```python
from build123d import *

# Parameters (mm, degrees)
SKETCH1_R           = 57.5
BOSS_EXTRUDE1_DEPTH = 4.5
SKETCH2_W           = 140
SKETCH2_H           = 70
BOSS_EXTRUDE2_DEPTH = 4.5
BOSS_EXTRUDE3_DEPTH = 4.5
SKETCH4_R           = 43
CUT_EXTRUDE1_DEPTH  = 5.5
SKETCH7_R           = 3.125
CUT_EXTRUDE8_DEPTH  = 5.5
LPATTERN1_COUNT     = 3
LPATTERN1_PITCH     = 20
CUT_EXTRUDE5_START  = -1
SKETCH5_R           = 2.125
CUT_EXTRUDE5_DEPTH  = 6.5
CIRPATTERN1_COUNT   = 12
SKETCH12_R          = 1.625
CUT_EXTRUDE17_DEPTH = 5.5
CIRPATTERN2_COUNT   = 4
SKETCH13_R          = 3.125
CUT_EXTRUDE18_DEPTH = 10
LPATTERN2_COUNT     = 3
LPATTERN2_PITCH     = 20


with BuildPart() as part:
    # Sketch1 → Boss-Extrude1 (new body)
    with BuildSketch(Plane(origin=(0, 0, 0), x_dir=(1, 0, 0), z_dir=(0, 1, 0))):
        Circle(SKETCH1_R)
    extrude(amount=BOSS_EXTRUDE1_DEPTH)

    # Sketch2 → Boss-Extrude2 (add)
    with BuildSketch(Plane(origin=(0, 0, 0), x_dir=(1, 0, 0), z_dir=(0, 1, 0))):
        with Locations((63.125798099, 0)):
            Rectangle(SKETCH2_W, SKETCH2_H)
    extrude(amount=BOSS_EXTRUDE2_DEPTH)

    # Sketch3 → Boss-Extrude3 (add)
    with BuildSketch(Plane(origin=(0, 0, 0), x_dir=(1, 0, 0), z_dir=(0, 1, 0))):
        Polygon((89.373258538, 35), (13.76852627, 55.827212758), (13.76852627, 13.558751548), align=None)
    extrude(amount=BOSS_EXTRUDE3_DEPTH)

    # Sketch4 → Cut-Extrude1 (cut, through all)
    with BuildSketch(Plane(origin=(0, 4.5, 0), x_dir=(1, 0, 0), z_dir=(0, 1, 0))):
        Circle(SKETCH4_R)
    extrude(amount=-CUT_EXTRUDE1_DEPTH, mode=Mode.SUBTRACT)

    # Sketch7 → Cut-Extrude8 (cut, through all)
    with BuildSketch(Plane(origin=(0, 4.5, 0), x_dir=(1, 0, 0), z_dir=(0, 1, 0))):
        with Locations((123.125798099, 15)):
            Circle(SKETCH7_R)
        with Locations((123.125798099, -15)):
            Circle(SKETCH7_R)
    cut_extrude8 = extrude(amount=-CUT_EXTRUDE8_DEPTH, mode=Mode.SUBTRACT)

    # LPattern1: Cut-Extrude8 ×3
    with Locations(*[(-i * LPATTERN1_PITCH, 0, 0) for i in range(1, LPATTERN1_COUNT)]):
        add(cut_extrude8, mode=Mode.SUBTRACT)

    # Sketch5 → Cut-Extrude5 (cut)
    with BuildSketch(Plane(origin=(0, 0, 0), x_dir=(1, 0, 0), z_dir=(0, 1, 0)).offset(CUT_EXTRUDE5_START)):
        with Locations((-51, 0)):
            Circle(SKETCH5_R)
    cut_extrude5 = extrude(amount=CUT_EXTRUDE5_DEPTH, mode=Mode.SUBTRACT)

    # CirPattern1: Cut-Extrude5 ×12 about axis
    cirpattern1_axis = Axis((0, 0, 0), (0, 1, 0))
    for i in range(1, CIRPATTERN1_COUNT):
        add(cut_extrude5.rotate(cirpattern1_axis, i * 360 / CIRPATTERN1_COUNT), mode=Mode.SUBTRACT)

    # Sketch12 → Cut-Extrude17 (cut, through all)
    with BuildSketch(Plane(origin=(0, 4.5, 0), x_dir=(1, 0, 0), z_dir=(0, 1, 0))):
        with Locations((-49.262217141, 13.1997713)):
            Circle(SKETCH12_R)
    cut_extrude17 = extrude(amount=-CUT_EXTRUDE17_DEPTH, mode=Mode.SUBTRACT)

    # CirPattern2: Cut-Extrude17 ×4 about axis
    cirpattern2_axis = Axis((0, 0, 0), (0, 1, 0))
    for i in range(1, CIRPATTERN2_COUNT):
        add(cut_extrude17.rotate(cirpattern2_axis, i * 360 / CIRPATTERN2_COUNT), mode=Mode.SUBTRACT)

    # Sketch13 → Cut-Extrude18 (cut)
    with BuildSketch(Plane(origin=(0, 4.5, 0), x_dir=(1, 0, 0), z_dir=(0, 1, 0))):
        with Locations((123.125798099, 0)):
            Circle(SKETCH13_R)
    cut_extrude18 = extrude(amount=-CUT_EXTRUDE18_DEPTH, mode=Mode.SUBTRACT)

    # LPattern2: Cut-Extrude18 ×3
    with Locations(*[(-i * LPATTERN2_PITCH, 0, 0) for i in range(1, LPATTERN2_COUNT)]):
        add(cut_extrude18, mode=Mode.SUBTRACT)


solid = part.part
```
Work out the finished part from the listing and answer in its coordinate system (mm). A direction names the side the tool comes from. Coordinates: 2 decimals unless noted, no trailing zeros. Write each loop counter-clockwise with the first axis right and the second up, starting at its lowest first coordinate (ties: lowest second). Pieces come first, ordered by that corner, then holes. Notation, with made-up numbers: (57.25, -22.75) - (96.25, -22.75) arc R27 cw to (96.25, 7.25) - close; hole circle Ø2 at (85.5, 66). An arc over 180 degrees is marked (long way). Answer as a JSON object with one key per item and string values.
Q1. Find section A-A (x = 0). Write down the section's boundary in (y, z) (3 decimals), plus the area to 4 significant figures.
Results list:
{"outline": "(0, -57.5) - (4.5, -57.5) - (4.5, -53.125) - (0, -53.125) - close; (0, -48.875) - (4.5, -48.875) - (4.5, -43) - (0, -43) - close; (0, 43) - (4.5, 43) - (4.5, 48.875) - (0, 48.875) - close; (0, 53.125) - (4.5, 53.125) - (4.5, 57.5) - (0, 57.5) - close", "area": "92.25 mm^2"}
Q2. Find section D-D (z = 39). Write down the section's boundary in (x, y), plus the area to 3 significant figures.
Results list:
{"outline": "(-42.25, 0) - (-18.11, 0) - (-18.11, 4.5) - (-42.25, 4.5) - close; (18.11, 0) - (42.25, 0) - (42.25, 4.5) - (18.11, 4.5) - close", "area": "217 mm^2"}
Q3. For a pull along X with two mould halves and no side action, classify faces 1 (the cylindrical face through (-26.481, 2.218, -46.053)), 2 (the cylindrical face through (-55.264, 2.218, 15.88)), 3 (the flat face through (58, 4.5, -1)), 4 (the cylindrical face through (45.96, 2.22, 26.64)) as pulls with the +X half, pulls with the -X half, needs draft (parallel to the pull), parting line crosses it, or undercut.
Results list:
{"face 1": "undercut", "face 2": "parting line crosses it", "face 3": "needs draft", "face 4": "undercut"}
Q4. Consider L1, parallel to Z at x = 124.5, y = 1.8; L2, parallel to X at y = 2.7, z = 43.5; L3, parallel to X at y = 2.7, z = -13.5. Determine where each line is inside the solid, lowest interval first. Write a range as from..to.
Results list:
{"L1": "z = -35..-17.81, -12.19..-2.81, 2.81..12.19, 17.81..35", "L2": "x = -37.6..-27.52, -23.48..23.48, 27.52..37.6", "L3": "x = -55.89..-50.86, -47.67..-40.83, 40.83..80.38, 85.87..100.38, 105.87..120.38, 125.87..133.13"}
Q5. Which of the six approach directions +Z, -Z, +X, -X, +Y, -Y give full straight-line access (tool end or side, diameter ignored) to faces 5 (the flat face through (89, 2, 35)), 6 (the flat face through (111, 2, -35)), 7 (the flat face through (58, 0, -1))?
Results list:
{"face 5": "+Z, +X, +Y, -Y", "face 6": "-Z, +X, +Y, -Y", "face 7": "+Z, -Z, +X, -X, -Y"}
Q6. Find section C-C (y = 1.5). State how many separate pieces and enclosed holes the cut face has, plus the area to 3 significant figures.
Results list:
{"separate pieces": "1", "enclosed holes": "26", "area": "10,000 mm^2"}
Q7. Given pin 1 Ø5.5 at (x, z) = (123.13, -15) entering from +Y; pin 2 Ø2 at (x, y) = (-1.5, 3.5) entering from -Z; pin 3 Ø1.5 at (x, y) = (55, 3.5) entering from +Z, each flat-ended and moving along its own axis, determine where each tip first touches the part or whether it passes through.
Results list:
{"pin 1": "passes through", "pin 2": "stops at z = -57.5", "pin 3": "stops at z = 35"}
Q8. Find section B-B (z = 0). Write down the section's boundary in (x, y) (3 decimals), plus the area to 3 significant figures.
Results list:
{"outline": "(-57.5, 0) - (-53.125, 0) - (-53.125, 4.5) - (-57.5, 4.5) - close; (-48.875, 0) - (-43, 0) - (-43, 4.5) - (-48.875, 4.5) - close; (43, 0) - (48.875, 0) - (48.875, 4.5) - (43, 4.5) - close; (53.125, 0) - (80.001, 0) - (80.001, 4.5) - (53.125, 4.5) - close; (86.251, 0) - (100.001, 0) - (100.001, 4.5) - (86.251, 4.5) - close; (106.251, 0) - (120.001, 0) - (120.001, 4.5) - (106.251, 4.5) - close; (126.251, 0) - (133.126, 0) - (133.126, 4.5) - (126.251, 4.5) - close", "area": "348 mm^2"}
